Check sheet for the modelled part. Datum: model origin and axes. Units: mm. Coordinates: 2 decimals unless noted, no trailing zeros. Loops run counter-clockwise (first coordinate to the right, second up) from the corner with the lowest first, then second, coordinate; pieces in that order, holes last.
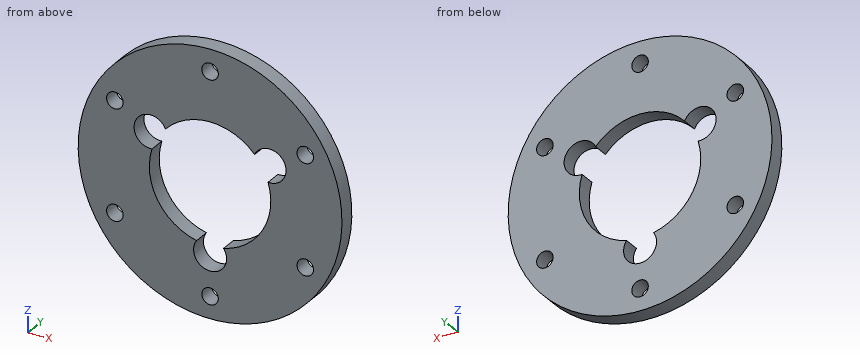
```python
from build123d import *

# Parameters (mm, degrees)
SKETCH_1_R          = 24
SKETCH_1_R_2        = 11.05
SKETCH_1_R_3        = 1.5
SKETCH_1_R_4        = 1.4
EXTRUDE_1_DEPTH     = 3
SKETCH_2_R          = 3
CUT_EXTRUDE_1_DEPTH = 10


with BuildPart() as part:
    # 草图1 → 凸台-拉伸1 (new body)
    with BuildSketch(Plane(origin=(0, 0, 0), x_dir=(1, 0, 0), z_dir=(0, 1, 0))):
        with Locations(Location((0, 0, 0), (0, 0, 270))):
            Circle(SKETCH_1_R)
        with Locations(Location((0, 0, 0), (0, 0, 270))):
            Circle(SKETCH_1_R_2, mode=Mode.SUBTRACT)
        with Locations(Location((0, 20, 0), (0, 0, 270))):
            Circle(SKETCH_1_R_3, mode=Mode.SUBTRACT)
        with Locations(Location((0, 12.5, 0), (0, 0, 270))):
            Circle(SKETCH_1_R_4, mode=Mode.SUBTRACT)
        with Locations(Location((17.320508076, 10, 0), (0, 0, 270))):
            Circle(SKETCH_1_R_3, mode=Mode.SUBTRACT)
        with Locations(Location((17.320508076, -10, 0), (0, 0, 270))):
            Circle(SKETCH_1_R_3, mode=Mode.SUBTRACT)
        with Locations(Location((0, -20, 0), (0, 0, 270))):
            Circle(SKETCH_1_R_3, mode=Mode.SUBTRACT)
        with Locations(Location((-17.320508076, -10, 0), (0, 0, 270))):
            Circle(SKETCH_1_R_3, mode=Mode.SUBTRACT)
        with Locations(Location((-17.320508076, 10, 0), (0, 0, 270))):
            Circle(SKETCH_1_R_3, mode=Mode.SUBTRACT)
        with Locations(Location((10.825317547, -6.25, 0), (0, 0, 270))):
            Circle(SKETCH_1_R_4, mode=Mode.SUBTRACT)
        with Locations(Location((-10.825317547, -6.25, 0), (0, 0, 270))):
            Circle(SKETCH_1_R_4, mode=Mode.SUBTRACT)
    extrude(amount=EXTRUDE_1_DEPTH)

    # 草图2 → 切除-拉伸1 (cut)
    with BuildSketch(Plane.XZ):
        with Locations((10.825317547, 6.25)):
            Circle(SKETCH_2_R)
        with Locations((-10.825317547, 6.25)):
            Circle(SKETCH_2_R)
        with Locations((0, -12.5)):
            Circle(SKETCH_2_R)
    extrude(amount=-CUT_EXTRUDE_1_DEPTH, mode=Mode.SUBTRACT)


solid = part.part
```
1) Section check B-B on x = 0. Enter the section's corners in (y, z), plus the area to 4 significant figures.
Answer sheet:
outline: (0, -24) - (3, -24) - (3, -21.5) - (0, -21.5) - close; (0, -18.5) - (3, -18.5) - (3, -15.5) - (0, -15.5) - close; (0, 11.05) - (3, 11.05) - (3, 18.5) - (0, 18.5) - close; (0, 21.5) - (3, 21.5) - (3, 24) - (0, 24) - close
area: 46.35 mm2
2) Scan lines: line 1 (X direction, y = 1.4, z = 9.5); line 2 (Z direction, x = -18, y = 0.25); line 3 (X direction, y = 0.9, z = 10). Record each from-to range of solid material in increasing order.
Answer sheet:
line 1: x = -22.04 to -18.73, -15.91 to -5.64, 5.64 to 15.91, 18.73 to 22.04
line 2: z = -15.87 to -11.34, -8.66 to 8.66, 11.34 to 15.87
line 3: x = -21.82 to -18.82, -15.82 to -4.7, 4.7 to 15.82, 18.82 to 21.82
3) Section check C-C on x = 10. Enter the section's corners in (y, z).
Answer sheet:
outline: (0, -21.82) - (3, -21.82) - (3, -4.7) - (0, -4.7) - close; (0, 9.13) - (3, 9.13) - (3, 21.82) - (0, 21.82) - close
4) Section check D-D on y = 2.5. Enter the section's corners in (x, z).
Answer sheet:
outline: circle Ø48 at (0, 0); hole circle Ø3 at (-17.32, -10); hole circle Ø3 at (-17.32, 10); hole (-10.56, 3.26) arc R11.05 ccw to (-2.45, -10.77) arc R3 ccw (long way) to (2.45, -10.77) arc R11.05 ccw to (10.56, 3.26) arc R3 ccw (long way) to (8.1, 7.51) arc R11.05 ccw to (-8.1, 7.51) arc R3 ccw (long way) to start; hole circle Ø3 at (0, -20); hole circle Ø3 at (0, 20); hole circle Ø3 at (17.32, -10); hole circle Ø3 at (17.32, 10)
5) Depth check by flat-ended pin: pin 1 (3.5 mm diameter, centred on x = 0, z = -12.5, fed in from +Y); pin 2 (1.5 mm diameter, centred on x = 6.5, y = 2, fed in from -Z). Enter the tip coordinate at first touch or a pass-through.
Answer sheet:
pin 1: passes through
pin 2: stops at z = -23.3
6) Section check A-A on z = 0. Enter the section's corners in (x, y).
Answer sheet:
outline: (-24, 0) - (-11.05, 0) - (-11.05, 3) - (-24, 3) - close; (11.05, 0) - (24, 0) - (24, 3) - (11.05, 3) - close
